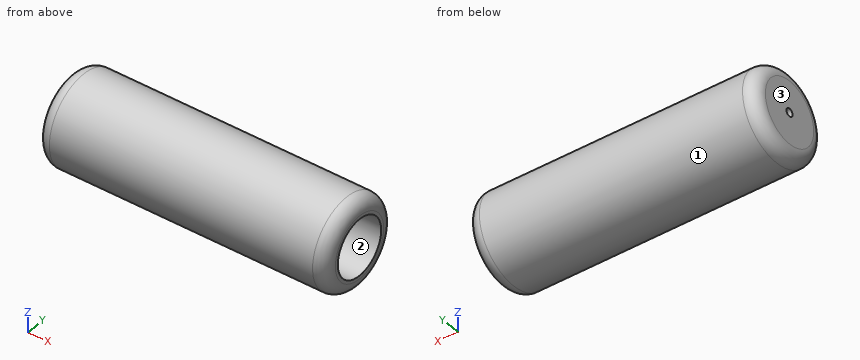
```python
from build123d import *

# Parameters (mm, degrees)
F2_R     = 5.08
F3_R     = 1.5792617016
F4_DEPTH = 25.4


with BuildPart() as f1:
    # F0 (on Front) → F1 (revolve)
    with BuildSketch(Plane.XZ):
        Polygon((-55.6552457488, -4.5627619832), (-55.6552457488, -22.0379619832), (57.8573542512, -22.0379619832), (57.8573542512, -15.6879619832), (-51.8719255924, -15.6879619832), (-51.6928457488, -4.5627619832), align=None)
    revolve(axis=Axis((-53.6740457488, 0, -4.5627619832), (1, 0, 0)))

    # F2
    f2_edges = [f1.edges().sort_by_distance(p)[0] for p in [
        (57.857354, 0, 12.912438),
        (-55.655246, 0, 12.912438),
    ]]
    fillet(f2_edges, radius=F2_R)

    # F3 (on face) → F4 (cut)
    with BuildSketch(Plane(origin=(-55.6552457488, 0, 0), x_dir=(0, -1, 0), z_dir=(-1, 0, 0))):
        with Locations((0, -4.5627619832)):
            Circle(F3_R)
    extrude(amount=-F4_DEPTH, mode=Mode.SUBTRACT)


solid = f1.part
```
Read the model definition and answer for the solid it produces. Units are mm, in the model's axes. Face numbers are marked on the shaded views. Give positions to 0.01 mm unless a question says otherwise; leave off trailing zeros. Order: outer loops, then holes, each group sorted by start corner. A loop starts at its lowest first (then second) coordinate and runs counter-clockwise, first axis right, second up. Notation, with made-up numbers: (53.25, -20) -> (102.25, -20) arc R10 cw to (102.25, -5) -> close; hole circle Ø6 at (-7.5, 53.25). An arc over 180 degrees is marked (long way). Write item = value, one per line.
1. A cutting plane is placed at A-A, the plane y = 0. Write down the section's boundary in (x, z).
Numbers:
outline = (-55.66, -16.96) arc R5.08 ccw to (-50.58, -22.04) -> (52.78, -22.04) arc R5.08 ccw to (57.86, -16.96) -> (57.86, -15.69) -> (-51.87, -15.69) -> (-51.72, -6.14) -> (-55.66, -6.14) -> close; (-55.66, -2.98) -> (-51.72, -2.98) -> (-51.87, 6.56) -> (57.86, 6.56) -> (57.86, 7.83) arc R5.08 ccw to (52.78, 12.91) -> (-50.58, 12.91) arc R5.08 ccw to (-55.66, 7.83) -> close
2. The mould has two halves that part along Z. Classify the marked faces 1, 2 and 3: +Z half, -Z half, draft (parallel to the pull), parting line (faces both ways), or undercut.
Numbers:
face_1 = parting line
face_2 = undercut
face_3 = draft
3. Given pin 1 (8 mm diameter, centred on x = -13, z = -11, fed in from -Y); pin 2 (13.5 mm diameter, centred on y = 0, z = -4.56, fed in from -X); pin 3 (3.5 mm diameter, centred on y = 0, z = -4.56, fed in from +X); pin 4 (5 mm diameter, centred on x = -4.5, y = 9, fed in from -Z), each flat-ended and moving along its own axis, determine where each tip first touches the part or whether it passes through.
Numbers:
pin_1 = -17.3
pin_2 = -55.66
pin_3 = -51.72
pin_4 = -20.78
4. Straight lines are drawn through the part: line 1 along Y through (x, z) = (-11.5, -4.5); line 2 along Y through (x, z) = (-48, 0); line 3 along Z through (x, y) = (39, 9.5). For each, find the intervals that lie inside material, in ascending order.
Numbers:
line_1 = -17.48 to -11.13, 11.13 to 17.48
line_2 = -16.87 to -10.15, 10.15 to 16.87
line_3 = -19.23 to -10.35, 1.23 to 10.1
5. A cutting plane is placed at B-B, the plane x = 33. Write down the section's boundary in (y, z), and give its area (3 significant figures).
Numbers:
outline = circle Ø34.95 at (0, -4.56); hole circle Ø22.25 at (0, -4.56)
area = 571 mm²
